Build history of the part. All positions in model axes, mm. Face numbers are marked on the shaded views. A direction names the side the tool comes from. Give positions to 0.01 mm unless a question says otherwise; leave off trailing zeros. Loops run counter-clockwise (first coordinate to the right, second up) from the corner with the lowest first, then second, coordinate; pieces in that order, holes last. Notation, with made-up numbers: M -27,72.25 L 9,72.25 A29 cw 9,97.25 Z; hole C 34,8 d10. An arc over 180 degrees is marked long. Answer as a JSON object with one key per item and string values. Group by question number.
1. Mould opens along Z. For the marked faces 1, 2 and 3 say: released by +Z, released by -Z, zero draft, split by the parting line, or undercut.
2. Drop flat-ended pins along their axis: pin 1 Ø5 at (x, y) = (1, 8) entering from -Z; pin 2 Ø1 at (y, z) = (-2.5, 4.5) entering from -X; pin 3 Ø6 at (y, z) = (9.5, 4) entering from +X. Give the stop position or say it passes through.
3. 3-axis set-ups, long thin cutter, end or side, ignore diameter. For the marked faces 4, 5, 6 and 7: which of +Z, -Z, +X, -X, +Y, -Y reach the whole face in a straight line?
4. Slice it at B-B (y = 4). List the corners of the cut face in (x, z), then the cut area to 3 significant figures.
from build123d import *
from build123d import SkipClean  # not in build123d's __all__

# Parameters (mm, degrees)
F1_DEPTH = 19.15
F2_R     = 2.75
F2_R_2   = 1.75
F3_DEPTH = 3
F5_DEPTH = 6
F6_W     = 10.1
F6_H     = 12.3
F7_DEPTH = 13.55


# Not quite as in the source:
# - after a boolean that leaves OpenCascade's solid faulty, fix() repairs it


with BuildPart() as f1:
    # F0 (on Front) → F1 (new body)
    with BuildSketch(Plane.XZ):
        Polygon((4.55, 8.05), (-4.55, 8.05), (-7.55, 3.55), (-7.55, -8.05), (7.55, -8.05), (7.55, 3.55), align=None)
    extrude(amount=F1_DEPTH)

    # F2 (on face) → F3 (join)
    with BuildSketch(Plane.XZ.offset(19.15)):
        with Locations((0, 2.95)):
            Circle(F2_R)
        with Locations((0, 2.95)):
            Circle(F2_R_2, mode=Mode.SUBTRACT)
    extrude(amount=F3_DEPTH)

    # F4 (on face) → F5 (cut)
    with BuildSketch(Plane.XZ.offset(19.15)):
        with BuildLine():
            Line((-7.55, -4.05), (-4.55, 0.5498131504))
            Line((-4.55, 0.5498131504), (-1.3422380888, 0.5498131504))
            ThreePointArc((-1.3422380888, 0.5498131504), (0, 5.7), (1.3422380888, 0.5498131504))
            Line((1.3422380888, 0.5498131504), (4.55, 0.5498131504))
            Line((4.55, 0.5498131504), (7.55, -4.05))
            Line((7.55, -4.05), (7.55, 3.55))
            Line((7.55, 3.55), (4.55, 8.05))
            Line((4.55, 8.05), (-4.55, 8.05))
            Line((-4.55, 8.05), (-7.55, 3.55))
            Line((-7.55, 3.55), (-7.55, -4.05))
        make_face()
    with SkipClean():  # cleaning this boolean's faces spoils the solid; the shape is the same uncleaned
        extrude(amount=-F5_DEPTH, mode=Mode.SUBTRACT)

    # F6 (on face) → F7 (join)
    with BuildSketch(Plane(origin=(0, 0, 0), x_dir=(-1, 0, 0), z_dir=(0, 1, 0))):
        with Locations((0, 3.1)):
            Rectangle(F6_W, F6_H)
    extrude(amount=F7_DEPTH)

    add(f1.part.fix(), mode=Mode.REPLACE)


solid = f1.part
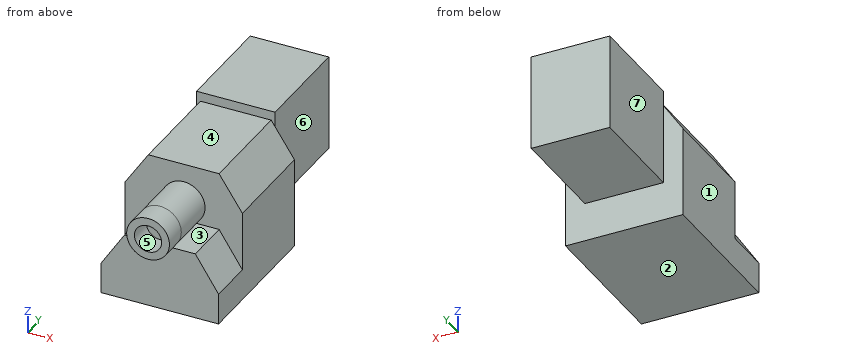
Established:
{
 "1": {"face 1": "zero draft", "face 2": "released by -Z", "face 3": "undercut"},
 "2": {"pin 1": "stops at z = -3.05", "pin 2": "stops at x = -7.25", "pin 3": "stops at x = 5.05"},
 "3": {"face 4": "+Z, +X, -X, -Y", "face 5": "-Y", "face 6": "+Z, -Z, +X, +Y", "face 7": "+Z, -Z, -X, +Y"},
 "4": {"outline": "M -5.05,-3.05 L 5.05,-3.05 L 5.05,9.25 L -5.05,9.25 Z", "area": "124 mm^2"}
}
